Read the model definition and answer for the solid it produces. Units are mm, in the model's axes. Face numbers are marked on the shaded views. A direction names the side the tool comes from. Give positions to 0.01 mm unless a question says otherwise; leave off trailing zeros. Write each loop counter-clockwise with the first axis right and the second up, starting at its lowest first coordinate (ties: lowest second). Pieces come first, ordered by that corner, then holes. Notation, with made-up numbers: (11.5, 84.5) -> (38.5, 84.5) arc R30 ccw to (38.5, 115.5) -> close; hole circle Ø4 at (31, 19). An arc over 180 degrees is marked (long way). Answer as CSV lines item,"result". Start each with the question number.
1. The part is cut by section C-C, the plane y = -4.25. Give the number of separate pieces and of enclosed holes in the cut face, and give its area (3 significant figures).
2. For a pull along X with two mould halves and no side action, classify the marked faces 1, 2 and 3 as pulls with the +X half, pulls with the -X half, needs draft (parallel to the pull), parting line crosses it, or undercut.
3. The part is cut by section D-D, the plane x = -2.75. Determine the outline of the cut face in (y, z).
4. Given pin 1 (1.5 mm diameter, centred on y = -5, z = 2, fed in from +X); pin 2 (2.5 mm diameter, centred on x = -8.11, y = -4, fed in from +Z); pin 3 (0.9 mm diameter, centred on y = -4, z = 3.5, fed in from -X), each flat-ended and moving along its own axis, determine where each tip first touches the part or whether it passes through.
5. The part is cut by section A-A, the plane y = -1.25. Determine the outline of the cut face in (x, z).
6. The part is cut by section B-B, the plane z = 1.75. Determine the outline of the cut face in (x, y), and give its area (3 significant figures).
7. A tool of negligible diameter and unlimited length cuts with its end or side. For the marked faces 4, 5, 6 and 7, from which of +Z, -Z, +X, -X, +Y, -Y can it reach the whole face along a straight path? Write none if from no direction.
8. Find the intervals of material crossed by line 1 (X direction, y = -4, z = 0.6); line 2 (X direction, y = -4, z = 1.35); line 3 (X direction, y = -2.5, z = 0.5), in increasing order.
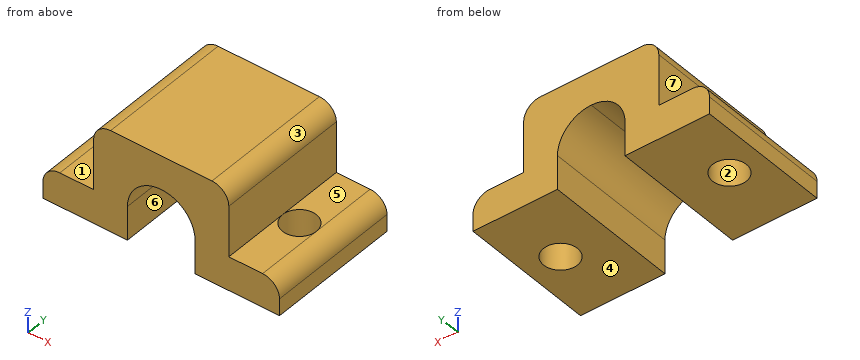
from build123d import *

# Parameters (mm, degrees)
F1_DEPTH = 8
F2_R     = 1
F3_DEPTH = 2
F4_R     = 1
F5_DEPTH = 2
F6_R     = 0.99999


# Not quite as in the source:
# - a fillet or chamfer is up to 0.001 mm smaller than in the source, because OpenCascade refuses the exact size


with BuildPart() as f1:
    # F0 (on Front) → F1 (new body)
    with BuildSketch(Plane.XZ):
        with BuildLine():
            Line((-10.1092506963, 2), (-10.1092506963, 0))
            Line((-10.1092506963, 0), (-5.1092506963, 0))
            Line((-5.1092506963, 0), (-5.1092506963, 2))
            ThreePointArc((-5.1092506963, 2), (-4.5234642587, 3.4142135624), (-3.1092506963, 4))
            ThreePointArc((-3.1092506963, 4), (-1.6950371339, 3.4142135624), (-1.1092506963, 2))
            Line((-1.1092506963, 2), (-1.1092506963, 0))
            Line((-1.1092506963, 0), (3.8907493037, 0))
            Line((3.8907493037, 0), (3.8907493037, 2))
            Line((3.8907493037, 2), (0.8907493037, 2))
            Line((0.8907493037, 2), (0.8907493037, 6))
            Line((0.8907493037, 6), (-7.1092506963, 6))
            Line((-7.1092506963, 6), (-7.1092506963, 2))
            Line((-7.1092506963, 2), (-10.1092506963, 2))
        make_face()
    extrude(amount=F1_DEPTH)

    # F2 (on face) → F3 (cut)
    with BuildSketch(Plane(origin=(0, 0, 0), x_dir=(1, 0, 0), z_dir=(0, 0, -1))):
        with Locations((-8.1092506963, 4)):
            Circle(F2_R)
    extrude(amount=-F3_DEPTH, mode=Mode.SUBTRACT)

    # F4 (on face) → F5 (cut)
    with BuildSketch(Plane(origin=(0, 0, 0), x_dir=(1, 0, 0), z_dir=(0, 0, -1))):
        with Locations((1.8907493037, 4)):
            Circle(F4_R)
    extrude(amount=-F5_DEPTH, mode=Mode.SUBTRACT)

    # F6 (radius 1 in the source; OpenCascade refuses exactly that, so slightly less here)
    f6_edges = [f1.edges().sort_by_distance(p)[0] for p in [
        (-10.109251, -4, 2),
        (-7.109251, -4, 6),
        (0.890749, -4, 6),
        (3.890749, -4, 2),
    ]]
    fillet(f6_edges, radius=F6_R)


solid = f1.part
Results found:
1,separate pieces,"3"
1,enclosed holes,"0"
1,area,"37.1 mm²"
2,face 1,"needs draft"
2,face 2,"undercut"
2,face 3,"pulls with the +X half"
3,outline,"(-8, 3.97) -> (0, 3.97) -> (0, 6) -> (-8, 6) -> close"
4,pin 1,"stops at x = 3.86"
4,pin 2,"stops at z = 5.66"
4,pin 3,"stops at x = -7.11"
5,outline,"(-10.11, 0) -> (-5.11, 0) -> (-5.11, 2) arc R2 cw to (-1.11, 2) -> (-1.11, 0) -> (3.89, 0) -> (3.89, 1) arc R1 ccw to (2.89, 2) -> (0.89, 2) -> (0.89, 5) arc R1 ccw to (-0.11, 6) -> (-6.11, 6) arc R1 ccw to (-7.11, 5) -> (-7.11, 2) -> (-9.11, 2) arc R1 ccw to (-10.11, 1) -> close"
6,outline,"(-9.77, -8) -> (-5.11, -8) -> (-5.11, 0) -> (-9.77, 0) -> close; (-1.11, -8) -> (3.55, -8) -> (3.55, 0) -> (-1.11, 0) -> close; hole circle Ø2 at (-8.11, -4); hole circle Ø2 at (1.89, -4)"
6,area,"68.3 mm²"
7,face 4,"-Z, +X, -X, +Y, -Y"
7,face 5,"+Z, +X, +Y, -Y"
7,face 6,"-Z, +Y, -Y"
7,face 7,"+Z, -X, +Y, -Y"
8,line 1,"x = -10.11 to -9.11, -7.11 to -5.11, -1.11 to 0.89, 2.89 to 3.89"
8,line 2,"x = -10.05 to -9.11, -7.11 to -5.11, -1.11 to 0.89, 2.89 to 3.83"
8,line 3,"x = -10.11 to -5.11, -1.11 to 3.89"
